Answer from the drawing. Dimensions are ordinates in mm from the lowest x, y and z of the part. A direction names the side the tool comes from. Coordinates: 2 decimals unless noted, no trailing zeros. Order: outer loops, then holes, each group sorted by start corner. A loop starts at its lowest first (then second) coordinate and runs counter-clockwise, first axis right, second up. Notation, with made-up numbers: (73, 87.25) -> (86, 87.25) arc R32 ccw to (86, 122.25) -> close; hole circle Ø5 at (6.5, -31). An arc over 180 degrees is marked (long way). Answer as a JSON object with one key per item and string values. Group by question number.
1) Consider L1, parallel to Z at x = 60, y = 39; L2, parallel to Y at x = 36, z = 20; L3, parallel to X at y = 43, z = 34. Determine where each line is inside the solid, lowest interval first.
2) Section C-C on z = 7 is taken. Determine the outline of the cut face in (x, y), and give its area (3 significant figures).
3) A tool of negligible diameter and unlimited length cuts with its end or side. For the marked faces 4, 5 and 6, from which of +Z, -Z, +X, -X, +Y, -Y can it reach the whole face along a straight path? Write none if from no direction.
4) Determine the mould class of the marked faces 1, 2 and 3 for opening direction Z: released by +Z, released by -Z, zero draft, split by the parting line, or undercut.
5) Section A-A on x = 36 is taken. Determine the outline of the cut face in (y, z), and give its area (3 significant figures).
6) Given pin 1 (2 mm diameter, centred on y = 60.5, z = 61, fed in from +X); pin 2 (12 mm diameter, centred on y = 39.5, z = 35, fed in from -X); pin 3 (6 mm diameter, centred on y = 44.5, z = 44.5, fed in from -X); pin 4 (19 mm diameter, centred on x = 36, y = 36, fed in from +Z), each flat-ended and moving along its own axis, determine where each tip first touches the part or whether it passes through.
7) Section B-B on y = 36 is taken. Determine the outline of the cut face in (x, z), and give its area (3 significant figures).
8) Section D-D on x = 13 is taken. Determine the outline of the cut face in (y, z), and give its area (3 significant figures).
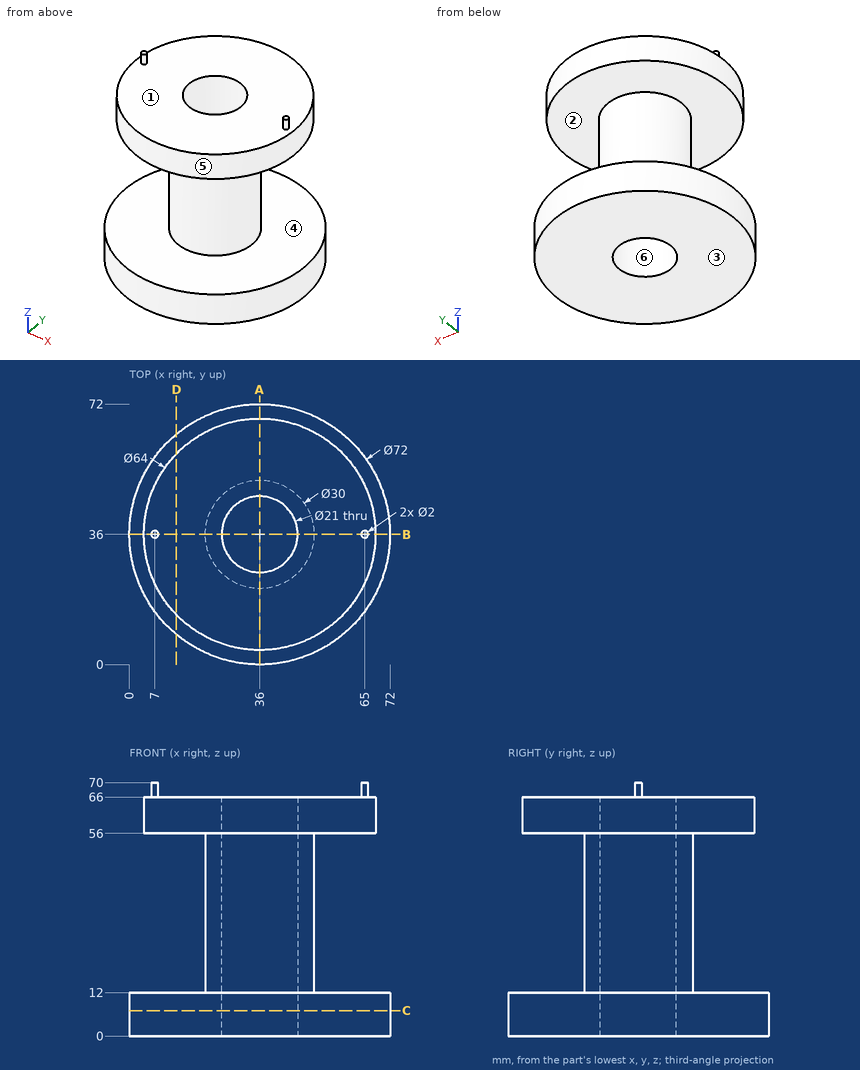
Worked answers:
{
 "1": {"L1": "z = 0 to 12, 56 to 66", "L2": "y = 21 to 25.5, 46.5 to 51", "L3": "x = 22.73 to 28.17, 43.83 to 49.27"},
 "2": {"outline": "circle Ø72 at (36, 36); hole circle Ø21 at (36, 36)", "area": "3,730 mm²"},
 "3": {"face 4": "none", "face 5": "+Z", "face 6": "+Z, -Z"},
 "4": {"face 1": "released by +Z", "face 2": "undercut", "face 3": "released by -Z"},
 "5": {"outline": "(0, 0) -> (25.5, 0) -> (25.5, 66) -> (4, 66) -> (4, 56) -> (21, 56) -> (21, 12) -> (0, 12) -> close; (46.5, 0) -> (72, 0) -> (72, 12) -> (51, 12) -> (51, 56) -> (68, 56) -> (68, 66) -> (46.5, 66) -> close", "area": "1,440 mm²"},
 "6": {"pin 1": "stops at x = 57.72", "pin 2": "stops at x = 21", "pin 3": "stops at x = 22.04", "pin 4": "passes through"},
 "7": {"outline": "(0, 0) -> (25.5, 0) -> (25.5, 66) -> (8, 66) -> (8, 70) -> (6, 70) -> (6, 66) -> (4, 66) -> (4, 56) -> (21, 56) -> (21, 12) -> (0, 12) -> close; (46.5, 0) -> (72, 0) -> (72, 12) -> (51, 12) -> (51, 56) -> (68, 56) -> (68, 66) -> (66, 66) -> (66, 70) -> (64, 70) -> (64, 66) -> (46.5, 66) -> close", "area": "1,450 mm²"},
 "8": {"outline": "(8.31, 0) -> (63.69, 0) -> (63.69, 12) -> (8.31, 12) -> close; (13.75, 56) -> (58.25, 56) -> (58.25, 66) -> (13.75, 66) -> close", "area": "1,110 mm²"}
}
